CAD build for the part. Positions are in the model's coordinates, mm. Face numbers are marked on the shaded views. A direction names the side the tool comes from. Give positions to 0.01 mm unless a question says otherwise; leave off trailing zeros. Write each loop counter-clockwise with the first axis right and the second up, starting at its lowest first coordinate (ties: lowest second). Pieces come first, ordered by that corner, then holes. Notation, with made-up numbers: (-36.75, 57) - (-23.75, 57) arc R6 ccw to (-23.75, 62) - close; hole circle Ø9 at (10, 76). An arc over 180 degrees is marked (long way). Put each result on its own line as item: value. Start each with the question number.
1. Tool access for the marked faces 5 and 6: list every direction of +Z, -Z, +X, -X, +Y, -Y with a clear straight run to the whole face (end or side of a thin tool).
2. Cut at A-A on z = -3.5. Give the number of separate pieces and of enclosed holes in the cut face, and give its area (3 significant figures).
3. Drop flat-ended pins along their axis: pin 1 (5 mm diameter, centred on x = 33, y = 6.5, fed in from +Z); pin 2 (3.5 mm diameter, centred on x = -3, y = 75, fed in from +Z). Give the stop position or say it passes through.
4. Cut at C-C on y = -24. List the corners of the cut face in (x, z), and give its area (3 significant figures).
5. Wall check: line 1 (Y direction, x = 35, z = -7.5); line 2 (X direction, y = 19, z = 11.5); line 3 (X direction, y = 29.5, z = -6). Give the ranges that are in metal, low to high.
6. Mould opens along X. For the marked faces 1, 2, 3 and 4 say: +X half, -X half, draft (parallel to the pull), parting line (faces both ways), or undercut.
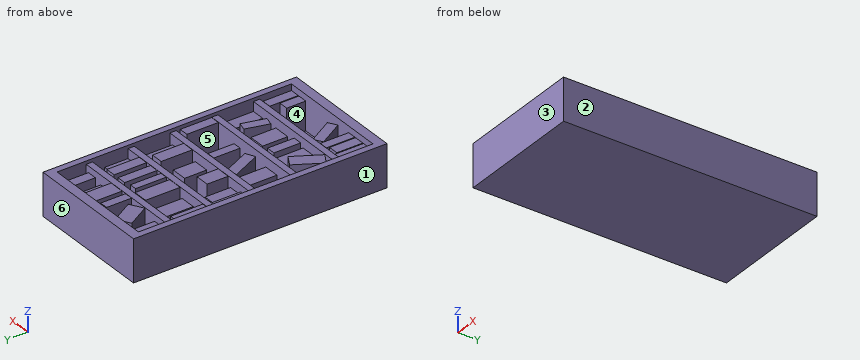
from build123d import *

# Parameters (mm, degrees)
SKETCH1_W           = 100
SKETCH1_H           = 33.333333334
BOSS_EXTRUDE1_DEPTH = 100
SKETCH2_W           = 90
SKETCH2_H           = 185
CUT_EXTRUDE1_DEPTH  = 27.5
SKETCH3_W           = 90
SKETCH3_H           = 5
BOSS_EXTRUDE2_DEPTH = 25
SKETCH4_W           = 7.5
SKETCH4_H           = 22.5
SKETCH4_H_2         = 15
SKETCH4_W_2         = 10
SKETCH4_W_3         = 8
SKETCH4_H_3         = 20.5
SKETCH4_W_4         = 6.75
BOSS_EXTRUDE5_DEPTH = 22.5
SKETCH5_W           = 10.245435458
SKETCH5_H           = 22.43939507
SKETCH5_W_2         = 12.999798951
SKETCH5_H_2         = 19.786374876
SKETCH5_W_3         = 12.203892893
SKETCH5_H_3         = 25.623019303
SKETCH5_W_4         = 7.857717283
SKETCH5_H_4         = 23.132751534
SKETCH5_W_5         = 12.203892892
SKETCH5_H_5         = 25
SKETCH5_W_6         = 6.632550485
SKETCH5_H_6         = 20.74503336
SKETCH5_W_7         = 10.346778757
SKETCH5_H_7         = 22.499597902
SKETCH5_W_8         = 12.601845922
SKETCH5_H_8         = 17.458859533
SKETCH5_W_9         = 8.489664621
SKETCH5_H_9         = 20.111879727
SKETCH5_H_10        = 18.417518017
SKETCH5_H_11        = 21.866444269
SKETCH5_W_10        = 8.75496664
SKETCH5_H_12        = 19.64147852
BOSS_EXTRUDE6_DEPTH = 17.5
SKETCH6_W           = 7.163154524
SKETCH6_H           = 21.112884973
SKETCH6_W_2         = 10.071772785
SKETCH6_H_2         = 24.928709858
SKETCH6_W_3         = 7.639556761
SKETCH6_H_3         = 23
SKETCH6_W_4         = 12.990267768
SKETCH6_H_4         = 19.731154058
BOSS_EXTRUDE7_DEPTH = 20
SKETCH7_W           = 7.443100334
SKETCH7_H           = 24.824572523
SKETCH7_W_2         = 11.141906558
SKETCH7_H_2         = 16.691268837
SKETCH7_W_3         = 9.597619028
SKETCH7_H_3         = 24.576310401
SKETCH7_W_4         = 7.222078614
SKETCH7_H_4         = 25.616891847
SKETCH7_W_5         = 11.567302571
SKETCH7_H_5         = 27.303769204
SKETCH7_W_6         = 5.774265567
SKETCH7_H_6         = 24.198791538
SKETCH7_W_7         = 7.404792338
SKETCH7_W_8         = 8.068151888
SKETCH7_W_9         = 12.035735356
SKETCH7_H_7         = 22.027016439
SKETCH7_W_10        = 6.605492776
SKETCH7_H_8         = 19.712859317
BOSS_EXTRUDE9_DEPTH = 24.75


with BuildPart() as part:
    # Sketch1 → Boss-Extrude1 (new body, symmetric)
    with BuildSketch(Plane(origin=(0, 0, 0), x_dir=(1, 0, 0), z_dir=(0, 1, 0))):
        Rectangle(SKETCH1_W, SKETCH1_H)
    extrude(amount=BOSS_EXTRUDE1_DEPTH, both=True)

    # Sketch2 → Cut-Extrude1 (cut)
    with BuildSketch(Plane.XY.offset(16.666666667)):
        Rectangle(SKETCH2_W, SKETCH2_H)
    extrude(amount=-CUT_EXTRUDE1_DEPTH, mode=Mode.SUBTRACT)

    # Sketch3 → Boss-Extrude2 (add)
    with BuildSketch(Plane.XY.offset(-10.833333333)):
        with Locations((0, -65)):
            Rectangle(SKETCH3_W, SKETCH3_H)
        with Locations((0, -32)):
            Rectangle(SKETCH3_W, SKETCH3_H)
        with Locations((0, 1)):
            Rectangle(SKETCH3_W, SKETCH3_H)
        with Locations((0, 34)):
            Rectangle(SKETCH3_W, SKETCH3_H)
        with Locations((0, 67)):
            Rectangle(SKETCH3_W, SKETCH3_H)
    extrude(amount=BOSS_EXTRUDE2_DEPTH)

    # Sketch4 → Boss-Extrude5 (add)
    with BuildSketch(Plane.XY.offset(-10.833333333)):
        with Locations((41.25, -81.25)):
            Rectangle(SKETCH4_W, SKETCH4_H)
        with Locations((33, -85)):
            Rectangle(SKETCH4_W, SKETCH4_H_2)
        with Locations((-39.5, -81.25)):
            Rectangle(SKETCH4_W_2, SKETCH4_H)
        with Locations((-29.7477, -82.25)):
            Rectangle(SKETCH4_W_3, SKETCH4_H_3)
        with Locations((-21.6227, -81.25)):
            Rectangle(SKETCH4_W_4, SKETCH4_H)
        Polygon((-17.9977, -72.764428415), (-6.7477, -92.25), (-0.252509472, -88.5), (-11.502509472, -69.014428415), align=None)
    extrude(amount=BOSS_EXTRUDE5_DEPTH)

    # Sketch5 → Boss-Extrude6 (add)
    with BuildSketch(Plane.XY.offset(-10.833333333)):
        with Locations((39.877282271, -51.280302465)):
            Rectangle(SKETCH5_W, SKETCH5_H)
        with Locations((13.663054, -52.606812562)):
            Rectangle(SKETCH5_W_2, SKETCH5_H_2)
        with Locations((-15.918121165, -49.688490349)):
            Rectangle(SKETCH5_W_3, SKETCH5_H_3)
        with Locations((-41.071141359, -17.933624233)):
            Rectangle(SKETCH5_W_4, SKETCH5_H_4)
        with Locations((-20.958859533, -17)):
            Rectangle(SKETCH5_W_5, SKETCH5_H_5)
        with Locations((16.846678233, -19.12748332)):
            Rectangle(SKETCH5_W_6, SKETCH5_H_6)
        with Locations((36.826610622, 14.749798951)):
            Rectangle(SKETCH5_W_7, SKETCH5_H_7)
        with Locations((10.545755271, 12.229429767)):
            Rectangle(SKETCH5_W_8, SKETCH5_H_8)
        with Locations((-26.264899922, 13.555939864)):
            Rectangle(SKETCH5_W_9, SKETCH5_H_9)
        with Locations((39.877282271, 45.708759009)):
            Rectangle(SKETCH5_W, SKETCH5_H_10)
        with Locations((-20.958859533, 47.433222134)):
            Rectangle(SKETCH5_W_5, SKETCH5_H_11)
        with Locations((24.540436795, 79.32073926)):
            Rectangle(SKETCH5_W_10, SKETCH5_H_12)
    extrude(amount=BOSS_EXTRUDE6_DEPTH)

    # Sketch6 → Boss-Extrude7 (add)
    with BuildSketch(Plane.XY.offset(-10.833333333)):
        with Locations((-3.581577262, -51.943557514)):
            Rectangle(SKETCH6_W, SKETCH6_H)
        Polygon((27.743083758, -42.568638898), (34.504564542, -44.380372214), (29.716412208, -62.25), (22.954931424, -60.438266684), align=None)
        Polygon((-14.606913087, -6.592305324), (-4.041456543, -29.25), (3.209005753, -25.869053906), (-7.35645079, -3.21135923), align=None)
        with Locations((-38.464113607, 15.964354929)):
            Rectangle(SKETCH6_W_2, SKETCH6_H_2)
        with Locations((38.68022162, 81)):
            Rectangle(SKETCH6_W_3, SKETCH6_H_3)
        with Locations((-37.004866116, 79.365577029)):
            Rectangle(SKETCH6_W_4, SKETCH6_H_4)
    extrude(amount=BOSS_EXTRUDE7_DEPTH)

    # Sketch7 → Boss-Extrude9 (add)
    with BuildSketch(Plane.XY.offset(-10.833333333)):
        Polygon((-22.270067611, -41.703177725), (-31.144265017, -36.579657463), (-43.006978388, -57.126479739), (-34.132780982, -62.25), align=None)
        with Locations((41.278449833, -17.087713739)):
            Rectangle(SKETCH7_W, SKETCH7_H)
        with Locations((-13.949114332, 11.845634419)):
            Rectangle(SKETCH7_W_2, SKETCH7_H_2)
        with Locations((24.961762989, 15.788155201)):
            Rectangle(SKETCH7_W_3, SKETCH7_H_3)
        with Locations((-41.388960693, 49.308445924)):
            Rectangle(SKETCH7_W_4, SKETCH7_H_4)
        with Locations((-6.788808075, 50.151884602)):
            Rectangle(SKETCH7_W_5, SKETCH7_H_5)
        with Locations((5.599653825, 48.599395769)):
            Rectangle(SKETCH7_W_6, SKETCH7_H_6)
        with Locations((16.460557306, 49.308445924)):
            Rectangle(SKETCH7_W_7, SKETCH7_H_4)
        with Locations((28.498967272, 49.308445924)):
            Rectangle(SKETCH7_W_8, SKETCH7_H_4)
        Polygon((-30.259732232, 87.284915382), (-20.135944116, 69.75), (-9.994868577, 75.604952692), (-20.118656693, 93.139868074), align=None)
        with Locations((11.35767736, 80.51350822)):
            Rectangle(SKETCH7_W_9, SKETCH7_H_7)
        with Locations((-1.87064299, 79.356429659)):
            Rectangle(SKETCH7_W_10, SKETCH7_H_8)
    extrude(amount=BOSS_EXTRUDE9_DEPTH)


solid = part.part
Report:
1. face 5: +Z
1. face 6: +Z, -Z, +X, -X, +Y
2. separate pieces: 5
2. enclosed holes: 7
2. area: 12,900 mm²
3. pin 1: stops at z = 6.67
3. pin 2: stops at z = 13.92
4. outline: (-50, -16.67) - (50, -16.67) - (50, 16.67) - (45, 16.67) - (45, 13.92) - (37.56, 13.92) - (37.56, -10.83) - (20.16, -10.83) - (20.16, 6.67) - (13.53, 6.67) - (13.53, -10.83) - (2.34, -10.83) - (2.34, 9.17) - (-6.49, 9.17) - (-6.49, -10.83) - (-14.86, -10.83) - (-14.86, 6.67) - (-27.06, 6.67) - (-27.06, -10.83) - (-37.14, -10.83) - (-37.14, 6.67) - (-45, 6.67) - (-45, 16.67) - (-50, 16.67) - close
4. area: 1,690 mm²
5. line 1: y = -100 to -77.5, -67.5 to -40.06, -34.5 to -29.5, -1.5 to 26, 31.5 to 54.92, 64.5 to 100
5. line 2: x = -50 to -45, -19.52 to -8.38, 20.16 to 29.76, 45 to 50
5. line 3: x = -50 to -45, 45 to 50
6. face 1: -X half
6. face 2: +X half
6. face 3: draft
6. face 4: undercut
